from build123d import *

# Parameters (mm, degrees)
BOSS_EXTRUDE1_DEPTH = 1.5
SKETCH2_R           = 22.5
BOSS_EXTRUDE4_DEPTH = 5
BOSS_EXTRUDE4_TAPER = 30
SKETCH3_R           = 7.5
BOSS_EXTRUDE5_DEPTH = 2
SKETCH4_R           = 9
BOSS_EXTRUDE7_DEPTH = 2
FILLET4_R           = 0.5
SKETCH5_R           = 1
CUT_EXTRUDE1_DEPTH  = 2


with BuildPart() as part:
    # Sketch1 → Boss-Extrude1 (new body)
    with BuildSketch(Plane.XY):
        with BuildLine():
            Line((-24, 24.5), (-24, -24.5))
            add(Edge.make_bspline(
                [(-24, -24.5), (-22.605605166, -29.952275609), (-14.106399585, -29.149385859), (-0.230857067, -26.321865732), (15.046005443, -29.389446711), (22.664200818, -29.845368103), (24, -24.5)],
                knots=[0, 0, 0, 0, 0.159886605, 0.492954102, 0.826021599, 1, 1, 1, 1], degree=3))
            Line((24, -24.5), (24, 24.5))
            add(Edge.make_bspline(
                [(-24, 24.5), (-22.605605166, 29.952275609), (-14.106399585, 29.149385859), (-0.230857067, 26.321865732), (15.046005443, 29.389446711), (22.664200818, 29.845368103), (24, 24.5)],
                knots=[0, 0, 0, 0, 0.159886605, 0.492954102, 0.826021599, 1, 1, 1, 1], degree=3))
        make_face()
    extrude(amount=BOSS_EXTRUDE1_DEPTH)

    # Sketch2 → Boss-Extrude4 (add)
    with BuildSketch(Plane.XY.offset(1.5)):
        Circle(SKETCH2_R)
    extrude(amount=BOSS_EXTRUDE4_DEPTH, taper=BOSS_EXTRUDE4_TAPER)

    # Sketch3 → Boss-Extrude5 (add)
    with BuildSketch(Plane.XY.offset(6.5)):
        Circle(SKETCH3_R)
    extrude(amount=BOSS_EXTRUDE5_DEPTH)

    # Sketch4 → Boss-Extrude7 (add)
    with BuildSketch(Plane.XY.offset(8.5)):
        Circle(SKETCH4_R)
    extrude(amount=BOSS_EXTRUDE7_DEPTH)

    # Fillet4
    fillet4_edges = [part.edges().sort_by_distance(p)[0] for p in [
        (-24, 0, 1.5),
        (0.007188855, 27.500047519, 1.5),
        (0.007188855, -27.500047519, 1.5),
        (24, 0, 1.5),
    ]]
    fillet(fillet4_edges, radius=FILLET4_R)

    # Sketch5 → Cut-Extrude1 (cut)
    with BuildSketch(Plane.XY.offset(1.5)):
        with Locations((18.5, -24.5)):
            Circle(SKETCH5_R)
        with Locations((-18.5, -24.5)):
            Circle(SKETCH5_R)
        with Locations((18.5, 24.5)):
            Circle(SKETCH5_R)
        with Locations((-18.5, 24.5)):
            Circle(SKETCH5_R)
    extrude(amount=-CUT_EXTRUDE1_DEPTH, mode=Mode.SUBTRACT)


solid = part.part
Input: part model. Units: mm. Frame: model coordinates. A direction names the side the tool comes from. Coordinates: 2 decimals unless noted, no trailing zeros. Write each loop counter-clockwise with the first axis right and the second up, starting at its lowest first coordinate (ties: lowest second). Pieces come first, ordered by that corner, then holes. Notation, with made-up numbers: M 42.5,34.25 L 67.5,34.25 A29 ccw 67.5,72.25 Z; hole C 16.25,11 d10. An arc over 180 degrees is marked long. Answer as a JSON object with one key per item and string values. Group by question number.
(1) Section A-A on y = 0. Output: boundary loops of the cut face in (x, z).
(2) Ray query, line 1 along Y through (x, z) = (-18.5, 0.85); line 2 along Z through (x, y) = (-21, -12.5); line 3 along Z through (x, y) = (10.5, 6). Return the intervals inside material, ascending. Write a range as [from, to].
(3) Section C-C on z = 9.75. Output: boundary loops of the cut face in (x, y), plus the area to 3 significant figures.
(4) Contact query for flat-ended pins moving along their axis: P1, Ø3, axis at y = 17, z = 5.5, coming from the -X side; P2, Ø1.5, axis at y = 16.5, z = 8, coming from the -X side; P3, Ø2.5, axis at x = 18.5, y = -24.5, coming from the +Z side; P4, Ø3, axis at y = 4, z = 9, coming from the -X side. Output: stop coordinate, or through.
(5) Set-up query: faces 4 (the face through (-11, 20, 1.5)), 5 (the face through (-7.493, 0.33, 7.486)), 6 (the face through (18.283, -25.476, 0.76)). Return all of +Z, -Z, +X, -X, +Y, -Y with unobstructed straight access to the full face (end or side cutting, diameter ignored); none if empty.
(6) Mould query, pull axis X, two halves, no side actions, for faces 1 (the face through (-1.172, 8.923, 9.486)), 2 (the face through (18.96, 23.61, 0.76)), 3 (the face through (-2, 7.4, 8.5)). Classes: pulls with the +X half, pulls with the -X half, needs draft (parallel to the pull), parting line crosses it, or undercut.
(7) Section B-B on x = 18.5. Give the number of separate pieces and of enclosed holes in the cut face, plus the area to 3 significant figures.
Result set:
{
 "1": {"outline": "M -24,0 L 24,0 L 24,1 A0.5 ccw 23.5,1.5 L 22.5,1.5 L 19.61,6.5 L 7.5,6.5 L 7.5,8.5 L 9,8.5 L 9,10.5 L -9,10.5 L -9,8.5 L -7.5,8.5 L -7.5,6.5 L -19.61,6.5 L -22.5,1.5 L -23.5,1.5 A0.5 ccw -24,1 Z"},
 "2": {"line 1": "y = [-29.48, -25.5], [-23.5, 23.5], [25.5, 29.48]", "line 2": "z = [0, 1.5]", "line 3": "z = [0, 6.5]"},
 "3": {"outline": "C 0,0 d18", "area": "254 mm2"},
 "4": {"P1": "stops at x = -13.39", "P2": "passes through", "P3": "stops at z = 1.5", "P4": "stops at x = -8.65"},
 "5": {"face 4": "+Z", "face 5": "none", "face 6": "+Z, -Z"},
 "6": {"face 1": "parting line crosses it", "face 2": "undercut", "face 3": "needs draft"},
 "7": {"separate pieces": "3", "enclosed holes": "0", "area": "182 mm2"}
}
